Read the model definition and answer for the solid it produces. Units are mm, in the model's axes. A direction names the side the tool comes from. Coordinates: 2 decimals unless noted, no trailing zeros. Write each loop counter-clockwise with the first axis right and the second up, starting at its lowest first coordinate (ties: lowest second). Pieces come first, ordered by that corner, then holes.
1) Each of these flat-tipped pins is pushed along its axis until it touches: pin 1 Ø3 at (x, y) = (1, 40) entering from +Z; pin 2 Ø1.5 at (y, z) = (38, -107) entering from -X. Where does it stop, or does it pass through?
2) Determine the mould class of faces 1 (the face through (0, 40, -110)), 2 (the face through (-13.25, 40, -107)), 3 (the face through (10.95, 41, -99)) for opening direction Z: +Z half, -Z half, draft (parallel to the pull), parting line (faces both ways), or undercut.
3) Find the intervals of material crossed by line 1 (X direction, y = 37.25, z = -102.25); line 2 (X direction, y = 36.75, z = -102); line 3 (X direction, y = 43.5, z = -104.75), in increasing order.
4) The part is cut by section B-B (z = -101.5). Give the number of separate pieces and of enclosed holes in the cut face, then the cut area to 3 significant figures.
5) The part is cut by section A-A (z = -97.25). Determine the outline of the cut face in (x, y).
6) The part is cut by section D-D (x = -2.5). Determine the outline of the cut face in (y, z).
7) Which of the six approach directions +Z, -Z, +X, -X, +Y, -Y give full straight-line access (tool end or side, diameter ignored) to faces 4 (the face through (13.25, 40, -108)), 5 (the face through (8.33, 42.5, -102.73)), 6 (the face through (-13, 40, -96.5)), 7 (the face through (-15.437, 40.676, -97.854))?
from build123d import *

# Parameters (mm, degrees)
SHAPE_DEPTH                   = 4
SHAPE_DEPTH_BACK              = 4
ESQUISSE19_R                  = 2.25
HOLEAXE_MOTOR_DEPTH           = 13
ESQUISSE20_R                  = 3.7
HOLEBEARING_MOTOR_DEPTH       = 3.2
ESQUISSE21_R                  = 2.2
ENTRETOISEBEARING_MOTOR_DEPTH = 1
EXT_MOTOR_START               = 3
ESQUISSE22_W                  = 10
ESQUISSE22_H                  = 8
ESQUISSE22_R                  = 2.25
EXT_MOTOR_DEPTH               = 3
ESQUISSE23_W                  = 3
ESQUISSE23_H                  = 7
HOLESCREWLESS_MOTOR_DEPTH     = 10
ESQUISSE24_W                  = 10
ESQUISSE24_H                  = 8
BOSS_EXTRU_1_DEPTH            = 3
ESQUISSE25_R                  = 1
REMOVE_HELPER_DEPTH           = 10


with BuildPart() as part:
    # Esquisse17 → Shape (new, two sides: drawn at the far end of the back side and taken through both)
    with BuildSketch(Plane(origin=(0, 40, 0), x_dir=(-1, 0, 0), z_dir=(0, -1, 0)).offset(-SHAPE_DEPTH_BACK)):
        Polygon((13.25, 105), (13.25, 95), (6.75, 95), (6.75, 105), (-6.75, 105), (-6.75, 95), (-13.25, 95), (-13.25, 105), (-13.25, 110), (13.25, 110), align=None)
    extrude(amount=SHAPE_DEPTH + SHAPE_DEPTH_BACK)

    # Esquisse19 → HoleAxe_motor (cut)
    with BuildSketch(Plane.ZY.offset(13.25)):
        with Locations((-100, 40)):
            Circle(ESQUISSE19_R)
    extrude(amount=-HOLEAXE_MOTOR_DEPTH, mode=Mode.SUBTRACT)

    # Esquisse20 → HoleBearing_motor (cut)
    with BuildSketch(Plane.ZY.offset(-6.75)):
        with Locations((-100, 40)):
            Circle(ESQUISSE20_R)
    holebearing_motor = extrude(amount=-HOLEBEARING_MOTOR_DEPTH, mode=Mode.SUBTRACT)

    # Symétrie3: HoleBearing_motor across plane
    add(holebearing_motor.mirror(Plane(origin=(0, 0, 0), x_dir=(0, 0, 1), z_dir=(1, 0, 0))), mode=Mode.SUBTRACT)

    # Esquisse21 → entretoiseBearing_motor (cut)
    with BuildSketch(Plane.ZY.offset(-9.95)):
        with Locations((-100, 40)):
            Circle(ESQUISSE21_R)
    extrude(amount=-ENTRETOISEBEARING_MOTOR_DEPTH, mode=Mode.SUBTRACT)

    # Esquisse22 → Ext_motor (add)
    with BuildSketch(Plane.ZY.offset(13.25).offset(EXT_MOTOR_START)):
        with Locations((-100, 40)):
            Rectangle(ESQUISSE22_W, ESQUISSE22_H)
        with Locations((-100, 40)):
            Circle(ESQUISSE22_R, mode=Mode.SUBTRACT)
    extrude(amount=-EXT_MOTOR_DEPTH)

    # Esquisse23 → HoleScrewLess_motor (cut)
    with BuildSketch(Plane(origin=(0, 44, 0), x_dir=(1, 0, 0), z_dir=(0, 1, 0))):
        with Locations((-13.1, 100)):
            Rectangle(ESQUISSE23_W, ESQUISSE23_H)
    extrude(amount=-HOLESCREWLESS_MOTOR_DEPTH, mode=Mode.SUBTRACT)

    # Esquisse24 → Boss.-Extru.1 (add)
    with BuildSketch(Plane(origin=(13.25, 0, 0), x_dir=(0, 0, -1), z_dir=(1, 0, 0))):
        with Locations((100, 40)):
            Rectangle(ESQUISSE24_W, ESQUISSE24_H)
    extrude(amount=BOSS_EXTRU_1_DEPTH)

    # Esquisse25 → Remove helper (cut)
    with BuildSketch(Plane.ZY.offset(-10.95)):
        with Locations((-100, 40)):
            Circle(ESQUISSE25_R)
    extrude(amount=-REMOVE_HELPER_DEPTH, mode=Mode.SUBTRACT)


solid = part.part
Reported:
1. pin 1: stops at z = -105
1. pin 2: stops at x = -13.25
2. face 1: -Z half
2. face 2: draft
2. face 3: undercut
3. line 1: x = -16.25 to -14.6, -11.6 to -9.95, 9.95 to 16.25
3. line 2: x = -16.25 to -14.6, -11.6 to -6.75, 6.75 to 16.25
3. line 3: x = -16.25 to -6.75, 6.75 to 16.25
4. separate pieces: 5
4. enclosed holes: 0
4. area: 70.4 mm2
5. outline: (-16.25, 36) - (-14.6, 36) - (-14.6, 44) - (-16.25, 44) - close; (-11.6, 36) - (-6.75, 36) - (-6.75, 37.52) - (-9.95, 37.52) - (-9.95, 42.48) - (-6.75, 42.48) - (-6.75, 44) - (-11.6, 44) - close; (6.75, 36) - (16.25, 36) - (16.25, 44) - (6.75, 44) - (6.75, 42.48) - (9.95, 42.48) - (9.95, 37.52) - (6.75, 37.52) - close
6. outline: (36, -110) - (44, -110) - (44, -105) - (36, -105) - close
7. face 4: -Z, +X, +Y, -Y
7. face 5: none
7. face 6: +Y, -Y
7. face 7: -X
